from build123d import *

# Parameters (mm, degrees)
EXTRUDE_1_DEPTH     = 4
EXTRUDE_START       = 2
EXTRUDE_2_DEPTH     = 2
EXTRUDE_3_DEPTH     = 2
SKETCH_4_R          = 1.6
CUT_EXTRUDE_1_DEPTH = 10
CUT_EXTRUDE_2_DEPTH = 3


with BuildPart() as part:
    # 草图1 → 凸台-拉伸1 (new body)
    with BuildSketch(Plane.XY):
        with BuildLine():
            Line((-35.40625, 64.537081934), (4.59375, 64.537081934))
            ThreePointArc((4.59375, 64.537081934), (10.957711031, 61.901042965), (13.59375, 55.537081934))
            Line((13.59375, 55.537081934), (13.59375, 15.537081934))
            ThreePointArc((13.59375, 15.537081934), (10.957711031, 9.173120903), (4.59375, 6.537081934))
            Line((4.59375, 6.537081934), (-35.40625, 6.537081934))
            ThreePointArc((-35.40625, 6.537081934), (-41.770211031, 9.173120903), (-44.40625, 15.537081934))
            Line((-44.40625, 15.537081934), (-44.40625, 55.537081934))
            ThreePointArc((-44.40625, 55.537081934), (-41.770211031, 61.901042965), (-35.40625, 64.537081934))
        make_face()
    extrude(amount=-EXTRUDE_1_DEPTH)

    # 草图2 → 凸台-拉伸2 (add)
    with BuildSketch(Plane.XY.offset(EXTRUDE_START)):
        with BuildLine():
            Line((13.59375, 15.537081934), (13.59375, 55.537081934))
            ThreePointArc((13.59375, 55.537081934), (10.957711031, 61.901042965), (4.59375, 64.537081934))
            Line((4.59375, 64.537081934), (-35.40625, 64.537081934))
            ThreePointArc((-35.40625, 64.537081934), (-41.770211031, 61.901042965), (-44.40625, 55.537081934))
            Line((-44.40625, 55.537081934), (-44.40625, 15.537081934))
            ThreePointArc((-44.40625, 15.537081934), (-41.770211031, 9.173120903), (-35.40625, 6.537081934))
            Line((-35.40625, 6.537081934), (4.59375, 6.537081934))
            ThreePointArc((4.59375, 6.537081934), (10.957711031, 9.173120903), (13.59375, 15.537081934))
        make_face()
        with BuildLine():
            Line((-35.40625, 63.537081934), (-25.40625, 63.537081934))
            Line((-25.40625, 63.537081934), (-25.40625, 45.537081934))
            Line((-25.40625, 45.537081934), (-43.40625, 45.537081934))
            Line((-43.40625, 45.537081934), (-43.40625, 55.537081934))
            ThreePointArc((-43.40625, 55.537081934), (-41.063104249, 61.193936184), (-35.40625, 63.537081934))
        make_face(mode=Mode.SUBTRACT)
        with BuildLine():
            Line((12.59375, 55.537081934), (12.59375, 45.537081934))
            Line((12.59375, 45.537081934), (-5.40625, 45.537081934))
            Line((-5.40625, 45.537081934), (-5.40625, 63.537081934))
            Line((-5.40625, 63.537081934), (4.59375, 63.537081934))
            ThreePointArc((4.59375, 63.537081934), (10.250604249, 61.193936184), (12.59375, 55.537081934))
        make_face(mode=Mode.SUBTRACT)
        with BuildLine():
            Line((-35.40625, 7.537081934), (-25.40625, 7.537081934))
            Line((-25.40625, 7.537081934), (-25.40625, 25.537081934))
            Line((-25.40625, 25.537081934), (-43.40625, 25.537081934))
            Line((-43.40625, 25.537081934), (-43.40625, 15.537081934))
            ThreePointArc((-43.40625, 15.537081934), (-41.063104249, 9.880227685), (-35.40625, 7.537081934))
        make_face(mode=Mode.SUBTRACT)
        with BuildLine():
            Line((-5.40625, 25.537081934), (12.59375, 25.537081934))
            Line((12.59375, 25.537081934), (12.59375, 15.537081934))
            ThreePointArc((12.59375, 15.537081934), (10.250604249, 9.880227685), (4.59375, 7.537081934))
            Line((4.59375, 7.537081934), (-5.40625, 7.537081934))
            Line((-5.40625, 7.537081934), (-5.40625, 25.537081934))
        make_face(mode=Mode.SUBTRACT)
    extrude(amount=-EXTRUDE_2_DEPTH)

    # 草图3 → 凸台-拉伸3 (add)
    with BuildSketch(Plane.XY.offset(2).offset(EXTRUDE_START)):
        with BuildLine():
            Line((13.59375, 15.537081934), (13.59375, 55.537081934))
            ThreePointArc((13.59375, 55.537081934), (10.957711031, 61.901042965), (4.59375, 64.537081934))
            Line((4.59375, 64.537081934), (-35.40625, 64.537081934))
            ThreePointArc((-35.40625, 64.537081934), (-41.770211031, 61.901042965), (-44.40625, 55.537081934))
            Line((-44.40625, 55.537081934), (-44.40625, 15.537081934))
            ThreePointArc((-44.40625, 15.537081934), (-41.770211031, 9.173120903), (-35.40625, 6.537081934))
            Line((-35.40625, 6.537081934), (4.59375, 6.537081934))
            ThreePointArc((4.59375, 6.537081934), (10.957711031, 9.173120903), (13.59375, 15.537081934))
        make_face()
        with BuildLine():
            Line((-43.40625, 55.537081934), (-43.40625, 45.537081934))
            Line((-43.40625, 45.537081934), (-43.40625, 25.537081934))
            Line((-43.40625, 25.537081934), (-43.40625, 15.537081934))
            ThreePointArc((-43.40625, 15.537081934), (-41.063104249, 9.880227685), (-35.40625, 7.537081934))
            Line((-35.40625, 7.537081934), (-25.40625, 7.537081934))
            Line((-25.40625, 7.537081934), (-5.40625, 7.537081934))
            Line((-5.40625, 7.537081934), (4.59375, 7.537081934))
            ThreePointArc((4.59375, 7.537081934), (10.250604249, 9.880227685), (12.59375, 15.537081934))
            Line((12.59375, 15.537081934), (12.59375, 25.537081934))
            Line((12.59375, 25.537081934), (12.59375, 45.537081934))
            Line((12.59375, 45.537081934), (12.59375, 55.537081934))
            ThreePointArc((12.59375, 55.537081934), (10.250604249, 61.193936184), (4.59375, 63.537081934))
            Line((4.59375, 63.537081934), (-5.40625, 63.537081934))
            Line((-5.40625, 63.537081934), (-25.40625, 63.537081934))
            Line((-25.40625, 63.537081934), (-35.40625, 63.537081934))
            ThreePointArc((-35.40625, 63.537081934), (-41.063104249, 61.193936184), (-43.40625, 55.537081934))
        make_face(mode=Mode.SUBTRACT)
    extrude(amount=-EXTRUDE_3_DEPTH)

    # 草图4 → 切除-拉伸1 (cut)
    with BuildSketch(Plane.XY.offset(2)):
        with Locations((-15.40625, 41.537081934)):
            Circle(SKETCH_4_R)
        with Locations((-15.40625, 29.537081934)):
            Circle(SKETCH_4_R)
        with Locations((4.59375, 35.537081934)):
            Circle(SKETCH_4_R)
        with Locations((-35.40625, 35.537081934)):
            Circle(SKETCH_4_R)
    extrude(amount=-CUT_EXTRUDE_1_DEPTH, mode=Mode.SUBTRACT)

    # 草图5 → 切除-拉伸2 (cut)
    with BuildSketch(Plane.XY.offset(2)):
        Polygon((-13.431907117, 44.024108978), (-16.572907158, 44.490426548), (-18.547250041, 42.003399505), (-17.380592883, 39.050054891), (-14.239592842, 38.58373732), (-12.265249959, 41.070764364), align=None)
        Polygon((1.418323519, 35.537081934), (3.00603676, 32.787081934), (6.18146324, 32.787081934), (7.769176481, 35.537081934), (6.18146324, 38.287081934), (3.00603676, 38.287081934), align=None)
        Polygon((-13.431907117, 27.050054891), (-12.265249959, 30.003399505), (-14.239592842, 32.490426548), (-17.380592883, 32.024108978), (-18.547250041, 29.070764364), (-16.572907158, 26.58373732), align=None)
        Polygon((-32.230823519, 35.537081934), (-33.81853676, 38.287081934), (-36.99396324, 38.287081934), (-38.581676481, 35.537081934), (-36.99396324, 32.787081934), (-33.81853676, 32.787081934), align=None)
    extrude(amount=-CUT_EXTRUDE_2_DEPTH, mode=Mode.SUBTRACT)


solid = part.part
For this review, take the finished solid that the model builds, in its own axes (mm). A direction names the side the tool comes from. Coordinates: 2 decimals unless noted, no trailing zeros. Order: outer loops, then holes, each group sorted by start corner. A loop starts at its lowest first (then second) coordinate and runs counter-clockwise, first axis right, second up. Notation, with made-up numbers: (-9.75, 58) - (19.25, 58) arc R14 cw to (19.25, 70) - close; hole circle Ø6 at (-37, 8). An arc over 180 degrees is marked (long way). Use one line per item in the form item = value.
Q1. Consider section B-B (x = -22). Give the boundary of the cut face in (y, z).
Checked values:
outline = (6.54, -4) - (64.54, -4) - (64.54, 4) - (63.54, 4) - (63.54, 2) - (7.54, 2) - (7.54, 4) - (6.54, 4) - close
Q2. Consider section A-A (z = 3). Give the boundary of the cut face in (x, y).
Checked values:
outline = (-44.41, 15.54) arc R9 ccw to (-35.41, 6.54) - (4.59, 6.54) arc R9 ccw to (13.59, 15.54) - (13.59, 55.54) arc R9 ccw to (4.59, 64.54) - (-35.41, 64.54) arc R9 ccw to (-44.41, 55.54) - close; hole (-43.41, 15.54) arc R8 ccw to (-35.41, 7.54) - (4.59, 7.54) arc R8 ccw to (12.59, 15.54) - (12.59, 55.54) arc R8 ccw to (4.59, 63.54) - (-35.41, 63.54) arc R8 ccw to (-43.41, 55.54) - close
Q3. For P1, Ø4.5, axis at x = -34.5, y = 35, coming from the +Z side; P2, Ø3, axis at x = -35.41, y = 35.54, coming from the +Z side; P3, Ø14.5, axis at x = -35.5, y = 55.5, coming from the +Z side; P4, Ø0.6, axis at y = 12, z = 1, coming from the +X side, all flat-tipped, find the tip position at first contact; note any pin that passes through.
Checked values:
P1 = 2
P2 = through
P3 = 0
P4 = 12.99
Q4. For probe 1 along Y at (x, z) = (-15.5, -3); probe 2 along X at (y, z) = (54.5, 1.5); probe 3 along X at (y, z) = (9, 0.5), list the stretches that pass through material, from the lowest coordinate up. Write a range as from..to.
Checked values:
probe_1 = 6.54..27.94, 31.13..39.94, 43.13..64.54
probe_2 = -44.41..-43.41, -25.41..-5.41, 12.59..13.59
probe_3 = -41.59..-40.02, -25.41..-5.41, 9.21..10.78
Q5. Consider section D-D (z = -3). Give the boundary of the cut face in (x, y), then the cut area to 3 significant figures.
Checked values:
outline = (-44.41, 15.54) arc R9 ccw to (-35.41, 6.54) - (4.59, 6.54) arc R9 ccw to (13.59, 15.54) - (13.59, 55.54) arc R9 ccw to (4.59, 64.54) - (-35.41, 64.54) arc R9 ccw to (-44.41, 55.54) - close; hole circle Ø3.2 at (-35.41, 35.54); hole circle Ø3.2 at (-15.41, 29.54); hole circle Ø3.2 at (-15.41, 41.54); hole circle Ø3.2 at (4.59, 35.54)
area = 3,260 mm2
Q6. For faces 5 (the flat face through (-35, 38.287, 1)), 6 (the flat face through (-44.406, 36, 0)), list the 3-axis set-ups (+Z, -Z, +X, -X, +Y, -Y) from which the entire face can be reached by the end or side of a thin tool; tool diameter is ignored.
Checked values:
face_5 = +Z
face_6 = +Z, -Z, -X, +Y, -Y
Q7. Draft analysis for pull direction X (two halves, no side actions). For faces 1 (the flat face through (-26, 64, 4)), 2 (the flat face through (13.594, 35, 0)), 3 (the flat face through (-37.8, 34.18, 0.52)), 4 (the cylindrical face through (-41.7, 61.97, 0.06)), state which applies: +X half, -X half, draft (parallel to the pull), parting line (faces both ways), or undercut.
Checked values:
face_1 = draft
face_2 = +X half
face_3 = undercut
face_4 = -X half
Q8. Consider section C-C (y = 22). Give the boundary of the cut face in (x, z).
Checked values:
outline = (-44.41, -4) - (13.59, -4) - (13.59, 4) - (12.59, 4) - (12.59, 0) - (-5.41, 0) - (-5.41, 2) - (-25.41, 2) - (-25.41, 0) - (-43.41, 0) - (-43.41, 4) - (-44.41, 4) - close
